```python
from build123d import *

# Parameters (mm, degrees)
PAD_DEPTH    = 5
PAD001_DEPTH = 1.6
PAD002_DEPTH = 4.5
FILLET_R     = 1.2


with BuildPart() as part:
    # Sketch → Pad (new body)
    with BuildSketch(Plane.XY):
        with BuildLine():
            ThreePointArc((1.6, -6.3), (0, 6.5), (-1.6, -6.3))
            Line((-1.6, -6.3), (-1.6, -5.262129))
            ThreePointArc((1.6, -5.262129), (0, 5.5), (-1.6, -5.262129))
            Line((1.6, -6.3), (1.6, -5.262129))
        make_face()
    extrude(amount=PAD_DEPTH)

    # Sketch001 (on Face6 of Pad) → Pad001 (join)
    with BuildSketch(Plane.XY.offset(5)):
        with BuildLine():
            ThreePointArc((1.6, -7.838367), (0, 8), (-1.6, -7.838367))
            Line((-1.6, -7.838367), (-1.6, -0.708872))
            ThreePointArc((1.6, -0.708872), (0, 1.75), (-1.6, -0.708872))
            Line((1.6, -7.838367), (1.6, -0.708872))
        make_face()
    extrude(amount=PAD001_DEPTH)

    # Sketch002 (on Face5 of Pad001) → Pad002 (join)
    with BuildSketch(Plane.XY.offset(6.6)):
        with BuildLine():
            ThreePointArc((1.6, -4.312772), (0, 4.6), (-1.6, -4.312772))
            Line((-1.6, -2.537716), (-1.6, -4.312772))
            ThreePointArc((1.6, -2.537716), (0, 3), (-1.6, -2.537716))
            Line((1.6, -2.537716), (1.6, -4.312772))
        make_face()
    extrude(amount=PAD002_DEPTH)

    # Fillet
    fillet_edges = [part.edges().sort_by_distance(p)[0] for p in [
        (0, 4.6, 6.6),
    ]]
    fillet(fillet_edges, radius=FILLET_R)


solid = part.part
```
Geometry check sheet. Reference: the model listing, model coordinates, mm. A direction names the side the tool comes from. Give positions to 0.01 mm unless a question says otherwise; leave off trailing zeros. Order: outer loops, then holes, each group sorted by start corner. A loop starts at its lowest first (then second) coordinate and runs counter-clockwise, first axis right, second up.
1. Release check for a two-part mould opening along X. For faces 1 (the face through (-1.3, 1.4, 5)), 2 (the face through (3, 5, 0)), 3 (the face through (0, 8, 6)) record: pulls with the +X half, pulls with the -X half, needs draft (parallel to the pull), parting line crosses it, or undercut.
2. Section check B-B, the plane z = 5.5. Enter the section's corners in (x, y), and give its area (3 significant figures).
3. Gauge pin test, flat ends, axial feed: pin 1 Ø5.5 at (x, y) = (1, 1) entering from -Z; pin 2 Ø1.5 at (y, z) = (-4.5, 4.5) entering from -X; pin 3 Ø4 at (y, z) = (-6, 5.5) entering from +X. Record the tip position at first contact, or that the pin passes through.
4. Access from +Z, -Z, +X, -X, +Y, -Y to the whole of each face (thin tool, end or side, straight path). Record for faces 4 (the face through (0, 3, 9)), 5 (the face through (0.219, 5.496, 2.465)), 6 (the face through (1.6, -5, 6)).
5. Thickness scan on L1, parallel to X at y = 0, z = 2.6; L2, parallel to X at y = 0, z = 5.7; L3, parallel to Z at x = -2.75, y = -6. Record the ranges inside material, lowest first.
6. Section check A-A, the plane x = 0. Enter the section's corners in (y, z).
7. Section check C-C, the plane z = 1.75. Enter the section's corners in (x, y), and give its area (3 significant figures).
Values follow:
1. face 1: undercut
1. face 2: needs draft
1. face 3: parting line crosses it
2. outline: (-1.6, -7.84) - (-1.6, -0.71) arc R1.75 cw (long way) to (1.6, -0.71) - (1.6, -7.84) arc R8 ccw (long way) to start
2. area: 171 mm2
3. pin 1: stops at z = 5
3. pin 2: stops at x = -6.96
3. pin 3: stops at x = 6.93
4. face 4: +Z
4. face 5: -Z
4. face 6: +Z, -Z, -Y
5. L1: x = -6.5 to -5.5, 5.5 to 6.5
5. L2: x = -8 to -1.75, 1.75 to 8
5. L3: z = 5 to 6.6
6. outline: (1.75, 5) - (5.5, 5) - (5.5, 0) - (6.5, 0) - (6.5, 5) - (8, 5) - (8, 6.6) - (5.8, 6.6) arc R1.2 cw to (4.6, 7.8) - (4.6, 11.1) - (3, 11.1) - (3, 6.6) - (1.75, 6.6) - close
7. outline: (-1.6, -6.3) - (-1.6, -5.26) arc R5.5 cw (long way) to (1.6, -5.26) - (1.6, -6.3) arc R6.5 ccw (long way) to start
7. area: 34.5 mm2
